Autodesk Inventor part; units mm, degrees
ref_plane "YZ Plane" through (0, 0, 0) normal (1, 0, 0) x (0, 1, 0)
ref_plane "XZ Plane" through (0, 0, 0) normal (0, 1, 0) x (-1, 0, 0)
ref_plane "XY Plane" through (0, 0, 0) normal (0, 0, 1) x (1, 0, 0)
sketch "Sketch1" plane through (0, 0, 0) normal (1, 0, 0) x (0, 1, 0)
  line L0 (-12.7, 12.7) -> (12.7, 12.7)
  line L1 (12.7, -12.7) -> (-12.7, -12.7)
  line L2 (12.7, 12.7) -> (25.4, 12.7)
  line L3 (25.4, 12.7) -> (25.4, -12.7)
  line L4 (25.4, -12.7) -> (12.7, -12.7)
  line L5 (-12.7, -12.7) -> (-25.4, -12.7)
  line L6 (-25.4, -12.7) -> (-25.4, 12.7)
  line L7 (-25.4, 12.7) -> (-12.7, 12.7)
  line L8 (22.86, -10.16) -> (22.86, 10.16)
  line L9 (22.86, 10.16) -> (12.7, 10.16)
  line L10 (12.7, 10.16) -> (-12.7, 10.16)
  line L11 (-12.7, 10.16) -> (-22.86, 10.16)
  line L12 (-22.86, 10.16) -> (-22.86, -10.16)
  line L13 (-22.86, -10.16) -> (-12.7, -10.16)
  line L14 (-12.7, -10.16) -> (12.7, -10.16)
  line L15 (12.7, -10.16) -> (22.86, -10.16)
  point P0 (0, 0)
  dimension "d1" = 25.4
  dimension "d14" = 25.4
  dimension "d15" = 50.8
  dimension "d16" = 12.7
  dimension "d17" = 2.54
extrude "Extrusion1" add sketch "Sketch1" along normal blind 1219.2
sketch "Sketch3" plane through (0, -25.4, 12.7) normal (0, 0, 1) x (1, 0, 0)
  line L0 (0, 25.4) -> (1219.2, 25.4) construction
  line L1 (1219.2, 0) -> (1219.2, 50.8) construction
  line L2 (0, 50.8) -> (1219.2, 50.8) construction
  line L3 (609.6, 50.8) -> (609.6, 0) construction
  line L4 (0, 0) -> (1219.2, 0) construction
  circle A0 centre (843.28, 25.4) radius 3.175
  circle A1 centre (375.92, 25.4) radius 3.175
  dimension "d20" = 6.35
  dimension "d21" = 233.68
  dimension "d22" = 233.68
extrude "Extrusion3" cut sketch "Sketch3" against normal through all
sketch "Sketch4" plane through (0, 25.4, 12.7) normal (0, 1, 0) x (1, 0, 0)
  line L0 (1219.2, 0) -> (1219.2, 25.4)
  line L1 (1219.2, 12.7) -> (0, 12.7) construction
  circle A0 centre (25.4, 12.7) radius 3.175
  circle A1 centre (1143, 12.7) radius 3.175
  line L2 (0, 25.4) -> (1219.2, 25.4) construction
  line L3 (609.6, 25.4) -> (609.6, 0) construction
  line L4 (0, 0) -> (1219.2, 0) construction
  line L5 (0, 25.4) -> (0, 0)
  circle A2 centre (762, 12.7) radius 3.175
  circle A3 centre (584.2, 12.7) radius 3.175
  dimension "d25" = 6.35
  dimension "d32" = 25.4
  dimension "d33" = 76.2
  dimension "d34" = 152.4
  dimension "d35" = 381
  dimension "d36" = 635
extrude "Extrusion4" cut sketch "Sketch4" against normal through all
equation "\"d22\" = d21"
properties part number "support-beam"
Geometry check sheet. Reference: the model listing, model coordinates, mm. A direction names the side the tool comes from. Coordinates: 2 decimals unless noted, no trailing zeros. Order: outer loops, then holes, each group sorted by start corner. A loop starts at its lowest first (then second) coordinate and runs counter-clockwise, first axis right, second up.
Item 1: Section check A-A (x = 687.5). Enter the section's corners in (y, z), plus the area to 3 significant figures.
Item 2: Depth check by flat-ended pin: pin 1 (10 mm diameter, centred on x = 25.4, z = 0, fed in from +Y); pin 2 (5.5 mm diameter, centred on x = 762, z = 0, fed in from +Y). Enter the tip coordinate at first touch or a pass-through.
Item 3: Tool access check on faces 1 (the flat face through (601, -22.86, 0)), 2 (the flat face through (601, 0, 12.7)). Record the directions out of +Z, -Z, +X, -X, +Y, -Y that give a thin tool (end or side, any length) a straight path to the whole face; none if there is none.
Item 4: Mould release check, pull along Y, two halves, no side actions. Record for faces 3 (the flat face through (601, 0, -10.16)), 4 (the flat face through (0, -0.1, 10.4)), 5 (the flat face through (601, -25.4, 0)): released by +Y, released by -Y, zero draft, split by the parting line, or undercut.
Item 5: Scan lines: line 1 along X through (y, z) = (-24.8, 0) (3 decimals); line 2 along Y through (x, z) = (179, 0.25); line 3 along Z through (x, y) = (758, 13). Record each from-to range of solid material in increasing order.
Check sheet entries:
1. outline: (-25.4, -12.7) - (25.4, -12.7) - (25.4, 12.7) - (-25.4, 12.7) - close; hole (-22.86, -10.16) - (22.86, -10.16) - (22.86, 10.16) - (-22.86, 10.16) - close
1. area: 361 mm2
2. pin 1: stops at y = 25.4
2. pin 2: passes through
3. face 1: +X, -X
3. face 2: +Z, +X, -X, +Y, -Y
4. face 3: undercut
4. face 4: zero draft
4. face 5: released by -Y
5. line 1: x = 0 to 22.225, 28.575 to 581.025, 587.375 to 758.825, 765.175 to 1139.825, 1146.175 to 1219.2
5. line 2: y = -25.4 to -22.86, 22.86 to 25.4
5. line 3: z = -12.7 to -10.16, 10.16 to 12.7
